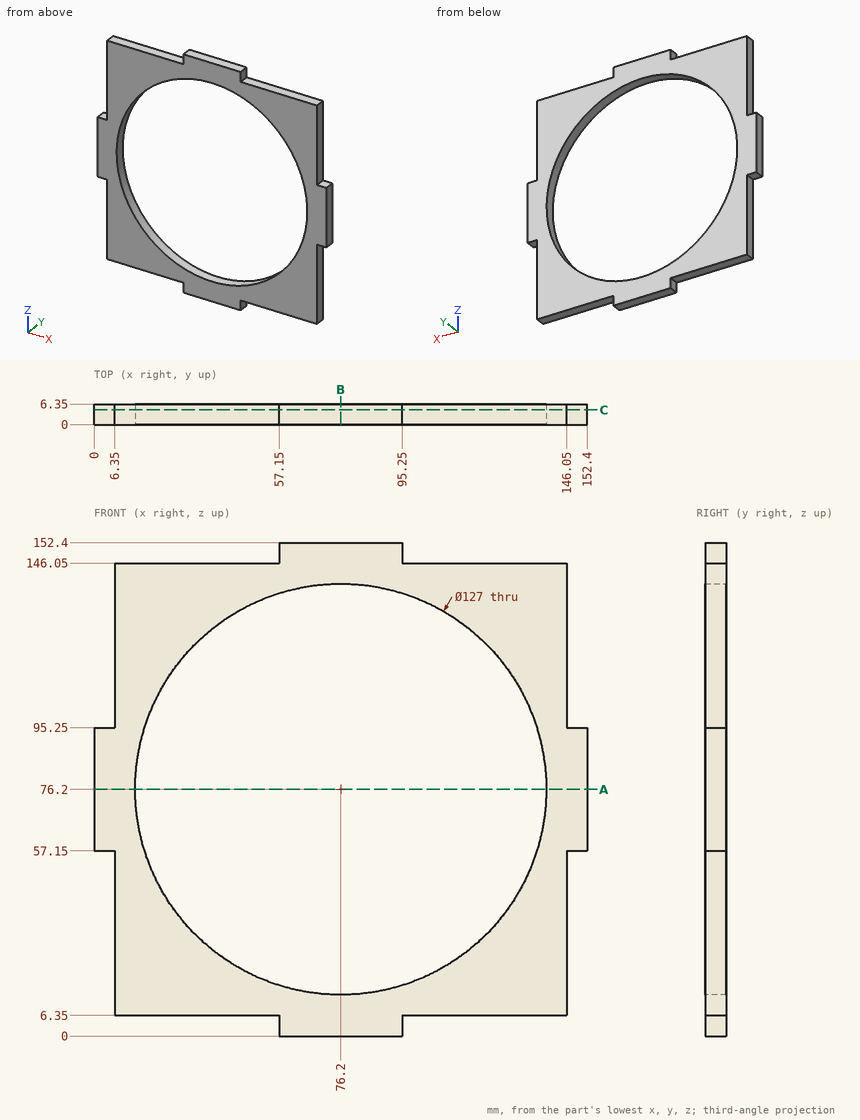
Verification items for this drawing (mm, ordinates from the low corner). Give positions to 0.01 mm unless a question says otherwise; leave off trailing zeros. Order: outer loops, then holes, each group sorted by start corner. A loop starts at its lowest first (then second) coordinate and runs counter-clockwise, first axis right, second up.
1) Gauge pin test, flat ends, axial feed: pin 1 (1 mm diameter, centred on x = 45, y = 2.5, fed in from +Z); pin 2 (3 mm diameter, centred on x = 53.5, y = 2.5, fed in from -Z); pin 3 (3 mm diameter, centred on y = 3.5, z = 148.5, fed in from -X). Record the tip position at first contact, or that the pin passes through.
Results are:
pin 1: stops at z = 146.05
pin 2: stops at z = 6.35
pin 3: stops at x = 57.15
2) Cross-section at B-B (x = 76.2). Record the boundary of the cut face in (y, z), then the cut area to 3 significant figures.
Results are:
outline: (0, 0) - (6.35, 0) - (6.35, 12.7) - (0, 12.7) - close; (0, 139.7) - (6.35, 139.7) - (6.35, 152.4) - (0, 152.4) - close
area: 161 mm2
3) Material ranges on probe 1 along X at (y, z) = (2.25, 76.2); probe 2 along X at (y, z) = (3.25, 144.5); probe 3 along Z at (x, y) = (38, 3.25), recorded low to high.
Results are:
probe 1: x = 0 to 12.7, 139.7 to 152.4
probe 2: x = 6.35 to 146.05
probe 3: z = 6.35 to 25.48, 126.92 to 146.05
4) Cross-section at C-C (y = 4.5). Record the boundary of the cut face in (x, z), then the cut area to 3 significant figures.
Results are:
outline: (0, 57.15) - (6.35, 57.15) - (6.35, 6.35) - (57.15, 6.35) - (57.15, 0) - (95.25, 0) - (95.25, 6.35) - (146.05, 6.35) - (146.05, 57.15) - (152.4, 57.15) - (152.4, 95.25) - (146.05, 95.25) - (146.05, 146.05) - (95.25, 146.05) - (95.25, 152.4) - (57.15, 152.4) - (57.15, 146.05) - (6.35, 146.05) - (6.35, 95.25) - (0, 95.25) - close; hole circle Ø127 at (76.2, 76.2)
area: 7,820 mm2
5) Cross-section at A-A (z = 76.2). Record the boundary of the cut face in (x, y), then the cut area to 3 significant figures.
Results are:
outline: (0, 0) - (12.7, 0) - (12.7, 6.35) - (0, 6.35) - close; (139.7, 0) - (152.4, 0) - (152.4, 6.35) - (139.7, 6.35) - close
area: 161 mm2
